For this review, take the finished solid that the model builds, in its own axes (mm). Coordinates: 2 decimals unless noted, no trailing zeros. Write each loop counter-clockwise with the first axis right and the second up, starting at its lowest first coordinate (ties: lowest second). Pieces come first, ordered by that corner, then holes.
```python
from build123d import *

# Parameters (mm, degrees)
SKETCH1_W           = 96
SKETCH1_H           = 66
SKETCH1_R           = 2.5
SKETCH1_R_2         = 1
BOSS_EXTRUDE1_DEPTH = 3
SKETCH2_W           = 14.25
SKETCH2_H           = 14.25
SKETCH2_W_2         = 3
SKETCH2_H_2         = 10
CUT_EXTRUDE1_DEPTH  = 3


with BuildPart() as part:
    # Sketch1 → Boss-Extrude1 (new body)
    with BuildSketch(Plane(origin=(0, 0, 0), x_dir=(1, 0, 0), z_dir=(0, 1, 0))):
        Rectangle(SKETCH1_W, SKETCH1_H)
        with Locations(Location((-39.75, 0, 0), (0, 0, 270))):
            Circle(SKETCH1_R, mode=Mode.SUBTRACT)
        with Locations(Location((39.75, 0, 0), (0, 0, 90))):
            Circle(SKETCH1_R, mode=Mode.SUBTRACT)
        with Locations(Location((-13.25, 29.75, 0), (0, 0, 270))):
            Circle(SKETCH1_R_2, mode=Mode.SUBTRACT)
        with Locations(Location((-13.25, 2, 0), (0, 0, 270))):
            Circle(SKETCH1_R_2, mode=Mode.SUBTRACT)
        with Locations(Location((13.25, 2, 0), (0, 0, 270))):
            Circle(SKETCH1_R_2, mode=Mode.SUBTRACT)
        with Locations(Location((13.25, 29.75, 0), (0, 0, 270))):
            Circle(SKETCH1_R_2, mode=Mode.SUBTRACT)
    extrude(amount=BOSS_EXTRUDE1_DEPTH)

    # Sketch2 → Cut-Extrude1 (cut)
    with BuildSketch(Plane(origin=(0, 3, 0), x_dir=(1, 0, 0), z_dir=(0, 1, 0))):
        with Locations((40.875, 25.875)):
            Rectangle(SKETCH2_W, SKETCH2_H)
        with Locations((-40.875, 25.875)):
            Rectangle(SKETCH2_W, SKETCH2_H)
        with Locations((40.875, -25.875)):
            Rectangle(SKETCH2_W, SKETCH2_H)
        with Locations((-40.875, -25.875)):
            Rectangle(SKETCH2_W, SKETCH2_H)
        with Locations((-25.5, -20)):
            Rectangle(SKETCH2_W_2, SKETCH2_H_2)
        with Locations((-25.5, 0)):
            Rectangle(SKETCH2_W_2, SKETCH2_H_2)
        with Locations((-25.5, 20)):
            Rectangle(SKETCH2_W_2, SKETCH2_H_2)
        with Locations((25.5, 20)):
            Rectangle(SKETCH2_W_2, SKETCH2_H_2)
        with Locations((25.5, -20)):
            Rectangle(SKETCH2_W_2, SKETCH2_H_2)
        with Locations((25.5, 0)):
            Rectangle(SKETCH2_W_2, SKETCH2_H_2)
    extrude(amount=-CUT_EXTRUDE1_DEPTH, mode=Mode.SUBTRACT)


solid = part.part
```
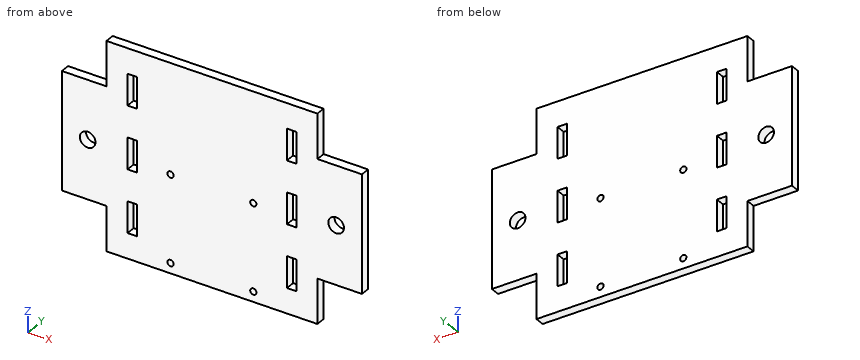
1) Consider section C-C (x = 39.75). Give the boundary of the cut face in (y, z), then the cut area to 3 significant figures.
2) Consider section D-D (y = 1.4). Count the separate pieces of the cut face and the enclosed holes in it, then the cut area to 3 significant figures.
3) Consider section A-A (x = -13.25). Give the boundary of the cut face in (y, z), then the cut area to 3 significant figures.
4) Consider section B-B (z = 4). Give the boundary of the cut face in (x, y).
5) Clearance check with flat-ended pins moving along their axes: P1, Ø1.5, axis at x = -41, y = 1, coming from the +Z side; P2, Ø1.5, axis at y = 2, z = 21.5, coming from the +X side. State where each tip first meets the part, or that it passes through.
6) For L1, parallel to X at y = 0.65, z = 20.5; L2, parallel to X at y = 0.9, z = 0; L3, parallel to X at y = 2.2, z = 16.5, list the stretches that pass through material, from the lowest coordinate up.
Results:
1. outline: (0, -18.75) - (3, -18.75) - (3, -2.5) - (0, -2.5) - close; (0, 2.5) - (3, 2.5) - (3, 18.75) - (0, 18.75) - close
1. area: 97.5 mm2
2. separate pieces: 1
2. enclosed holes: 12
2. area: 5,290 mm2
3. outline: (0, -33) - (3, -33) - (3, -30.75) - (0, -30.75) - close; (0, -28.75) - (3, -28.75) - (3, -3) - (0, -3) - close; (0, -1) - (3, -1) - (3, 33) - (0, 33) - close
3. area: 186 mm2
4. outline: (-48, 0) - (-27, 0) - (-27, 3) - (-48, 3) - close; (-24, 0) - (24, 0) - (24, 3) - (-24, 3) - close; (27, 0) - (48, 0) - (48, 3) - (27, 3) - close
5. P1: stops at z = 18.75
5. P2: stops at x = 33.75
6. L1: x = -33.75 to -27, -24 to 24, 27 to 33.75
6. L2: x = -48 to -42.25, -37.25 to -27, -24 to 24, 27 to 37.25, 42.25 to 48
6. L3: x = -48 to -27, -24 to 24, 27 to 48
